Answer from the drawing. Dimensions are ordinates in mm from the lowest x, y and z of the part. A direction names the side the tool comes from. Give positions to 0.01 mm unless a question says otherwise; leave off trailing zeros. Write each loop counter-clockwise with the first axis right and the second up, starting at its lowest first coordinate (ties: lowest second). Pieces come first, ordered by that corner, then holes.
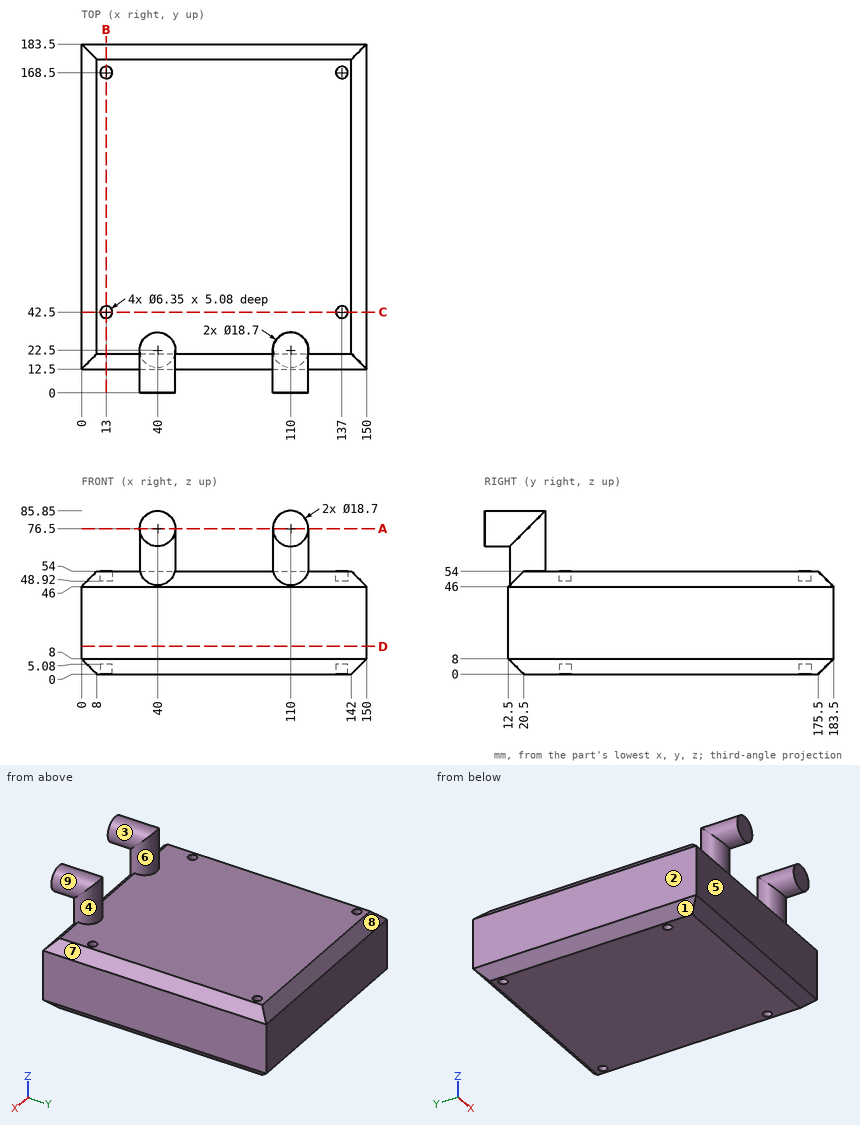
Item 1: Each of these flat-tipped pins is pushed along its axis until it touches: P1, Ø8.5, axis at x = 13, y = 42.5, coming from the +Z side; P2, Ø5, axis at x = 13, y = 168.5, coming from the -Z side; P3, Ø1.9, axis at x = 135.5, y = 167, coming from the +Z side. Where does it stop, or does it pass through?
Conclusion:
P1: stops at z = 54
P2: stops at z = 5.08
P3: stops at z = 48.92
Item 2: A cutting plane is placed at A-A, the plane z = 76.5. Give the vertices of the cut face in (x, y).
Conclusion:
outline: (30.65, 0) - (49.35, 0) - (49.35, 22.5) arc R9.35 ccw to (30.65, 22.5) - close; (100.65, 0) - (119.35, 0) - (119.35, 22.5) arc R9.35 ccw to (100.65, 22.5) - close
Item 3: A cutting plane is placed at D-D, the plane z = 14.5. Give the vertices of the cut face in (x, y), plus the area to 4 significant figures.
Conclusion:
outline: (0, 12.5) - (150, 12.5) - (150, 183.5) - (0, 183.5) - close
area: 25,650 mm2
Item 4: A cutting plane is placed at C-C, the plane y = 42.5. Give the vertices of the cut face in (x, z) (3 decimals).
Conclusion:
outline: (0, 8) - (8, 0) - (9.825, 0) - (9.825, 5.08) - (16.175, 5.08) - (16.175, 0) - (133.825, 0) - (133.825, 5.08) - (140.175, 5.08) - (140.175, 0) - (142, 0) - (150, 8) - (150, 46) - (142, 54) - (140.175, 54) - (140.175, 48.92) - (133.825, 48.92) - (133.825, 54) - (16.175, 54) - (16.175, 48.92) - (9.825, 48.92) - (9.825, 54) - (8, 54) - (0, 46) - close
Item 5: Consider probe 1 along X at (y, z) = (168.5, 1.5) (3 decimals); probe 2 along X at (y, z) = (42, 2); probe 3 along Y at (x, z) = (137, 52) (3 decimals). Determine where each line is inside the solid, lowest interval first.
Conclusion:
probe 1: x = 6.5 to 9.825, 16.175 to 133.825, 140.175 to 143.5
probe 2: x = 6 to 9.86, 16.14 to 133.86, 140.14 to 144
probe 3: y = 18.5 to 39.325, 45.675 to 165.325, 171.675 to 177.5
Item 6: A cutting plane is placed at B-B, the plane x = 13. Give the vertices of the cut face in (y, z) (3 decimals), plus the area to 3 significant figures.
Conclusion:
outline: (12.5, 8) - (20.5, 0) - (39.325, 0) - (39.325, 5.08) - (45.675, 5.08) - (45.675, 0) - (165.325, 0) - (165.325, 5.08) - (171.675, 5.08) - (171.675, 0) - (175.5, 0) - (183.5, 8) - (183.5, 46) - (175.5, 54) - (171.675, 54) - (171.675, 48.92) - (165.325, 48.92) - (165.325, 54) - (45.675, 54) - (45.675, 48.92) - (39.325, 48.92) - (39.325, 54) - (20.5, 54) - (12.5, 46) - close
area: 8,980 mm2
Item 7: Which of the six approach directions +Z, -Z, +X, -X, +Y, -Y give full straight-line access (tool end or side, diameter ignored) to the marked faces 1, 2, 3, 4 and 5?
Conclusion:
face 1: -Z, -X, +Y, -Y
face 2: +Z, -Z, -X, +Y, -Y
face 3: -Y
face 4: none
face 5: -Z, +X, -X, -Y
Item 8: Determine the mould class of the marked faces 6, 7, 8 and 9 for opening direction X: pulls with the +X half, pulls with the -X half, needs draft (parallel to the pull), parting line crosses it, or undercut.
Conclusion:
face 6: undercut
face 7: pulls with the +X half
face 8: needs draft
face 9: undercut
